```python
from build123d import *

# Parameters (mm, degrees)
SKIZZE1_W                                            = 33
SKIZZE1_H                                            = 20
SKIZZE1_W_2                                          = 13
SKIZZE1_H_2                                          = 13
AUFSATZ_LINEAR_AUSTRAGEN1_DEPTH                      = 10
STIRNSENKUNG_F_R_M4_ZYLINDERSCHRAUBE_MIT_D           = 4.5
STIRNSENKUNG_F_R_M4_ZYLINDERSCHRAUBE_MIT_CBORE_D     = 8
STIRNSENKUNG_F_R_M4_ZYLINDERSCHRAUBE_MIT_CBORE_DEPTH = 4.4
SKIZZE8_R                                            = 2.25
SCHNITT_LINEAR_AUSTRAGEN1_DEPTH                      = 11
M5_GEWINDEBOHRUNG1_D                                 = 4.2


with BuildPart() as part:
    # Skizze1 → Aufsatz-Linear austragen1 (new body)
    with BuildSketch(Plane.XY):
        Rectangle(SKIZZE1_W, SKIZZE1_H)
        Rectangle(SKIZZE1_W_2, SKIZZE1_H_2, mode=Mode.SUBTRACT)
    extrude(amount=AUFSATZ_LINEAR_AUSTRAGEN1_DEPTH)

    # Stirnsenkung für M4 Zylinderschraube mit Innensechskant1 (through all)
    with Locations(Plane.XY.offset(10)):
        with Locations((-11.5, 0)):
            CounterBoreHole(STIRNSENKUNG_F_R_M4_ZYLINDERSCHRAUBE_MIT_D / 2, STIRNSENKUNG_F_R_M4_ZYLINDERSCHRAUBE_MIT_CBORE_D / 2, STIRNSENKUNG_F_R_M4_ZYLINDERSCHRAUBE_MIT_CBORE_DEPTH)

    # Skizze8 → Schnitt-Linear austragen1 (cut, through all)
    with BuildSketch(Plane.XY.offset(10)):
        with Locations((-6.5, 6.5)):
            Circle(SKIZZE8_R)
        with Locations((-6.5, -6.5)):
            Circle(SKIZZE8_R)
        with Locations((6.5, -6.5)):
            Circle(SKIZZE8_R)
        with Locations((6.5, 6.5)):
            Circle(SKIZZE8_R)
    extrude(amount=-SCHNITT_LINEAR_AUSTRAGEN1_DEPTH, mode=Mode.SUBTRACT)

    # M5 Gewindebohrung1 (through all)
    with Locations(Plane.XY.offset(10)):
        with Locations((11.5, 0)):
            Hole(M5_GEWINDEBOHRUNG1_D / 2)


solid = part.part
```
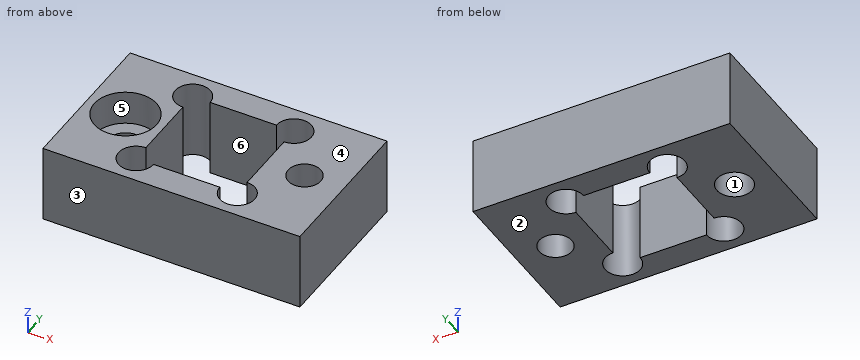
Model file for the job. Use its own axes, mm. Face numbers are marked on the shaded views. A direction names the side the tool comes from. Coordinates: 2 decimals unless noted, no trailing zeros. Order: outer loops, then holes, each group sorted by start corner. A loop starts at its lowest first (then second) coordinate and runs counter-clockwise, first axis right, second up. Notation, with made-up numbers: (22, -0.5) -> (48, -0.5) arc R8 cw to (48, 12.5) -> close; hole circle Ø10 at (-8, 31.5). An arc over 180 degrees is marked (long way). Answer as a JSON object with one key per item and string values. Group by question number.
1) Cut at A-A, the plane x = 11.5. Write the cut outline in (y, z).
2) Drill centre lines: L1, parallel to Y at x = 3.5, z = 0.5; L2, parallel to Y at x = 7.5, z = 5.5; L3, parallel to X at y = -7, z = 9.75. Where is each one in solid material? Low to high.
3) Cut at C-C, the plane y = 3.25. Write the cut outline in (x, z).
4) Flat gauge pins, fed straight in: pin 1 (2.5 mm diameter, centred on x = -12.5, y = -1.5, fed in from +Z); pin 2 (4 mm diameter, centred on x = 6.5, y = -6.5, fed in from -Z). Where does each tip first touch, or does it go through?
5) Which spindle directions (+Z, -Z, +X, -X, +Y, -Y) get a long thin tool onto all of the face, cutting with end or side? Do the marked faces 4, 5 and 6. Say none if no direction does.
6) Pull direction Y, two halves, no side cores. Call the marked faces 1, 2 and 3: +Y half, -Y half, draft (parallel to the pull), parting line (faces both ways), or undercut.
7) Cut at B-B, the plane z = 3.5. Write the cut outline in (x, y), then the cut area to 3 significant figures.
8) Cut at D-D, the plane x = -7. Write the cut outline in (y, z).
Check values:
{
 "1": {"outline": "(-10, 0) -> (-2.1, 0) -> (-2.1, 10) -> (-10, 10) -> close; (2.1, 0) -> (10, 0) -> (10, 10) -> (2.1, 10) -> close"},
 "2": {"L1": "y = -10 to -6.5, 6.5 to 10", "L2": "y = -10 to -8.52, -4.48 to 4.48, 8.52 to 10", "L3": "x = -16.5 to -8.69, -4.31 to 4.31, 8.69 to 16.5"},
 "3": {"outline": "(-16.5, 0) -> (-6.5, 0) -> (-6.5, 10) -> (-9.17, 10) -> (-9.17, 5.6) -> (-13.83, 5.6) -> (-13.83, 10) -> (-16.5, 10) -> close; (6.5, 0) -> (16.5, 0) -> (16.5, 10) -> (6.5, 10) -> close"},
 "4": {"pin 1": "stops at z = 5.6", "pin 2": "passes through"},
 "5": {"face 4": "+Z, +X, -X, +Y, -Y", "face 5": "+Z", "face 6": "+Z, -Z"},
 "6": {"face 1": "undercut", "face 2": "draft", "face 3": "-Y half"},
 "7": {"outline": "(-16.5, -10) -> (16.5, -10) -> (16.5, 10) -> (-16.5, 10) -> close; hole circle Ø4.5 at (-11.5, 0); hole (-6.5, -4.25) arc R2.25 ccw (long way) to (-4.25, -6.5) -> (4.25, -6.5) arc R2.25 ccw (long way) to (6.5, -4.25) -> (6.5, 4.25) arc R2.25 ccw (long way) to (4.25, 6.5) -> (-4.25, 6.5) arc R2.25 ccw (long way) to (-6.5, 4.25) -> close; hole circle Ø4.2 at (11.5, 0)", "area": "414 mm²"},
 "8": {"outline": "(-10, 0) -> (-8.69, 0) -> (-8.69, 10) -> (-10, 10) -> close; (-4.31, 0) -> (4.31, 0) -> (4.31, 10) -> (-4.31, 10) -> close; (8.69, 0) -> (10, 0) -> (10, 10) -> (8.69, 10) -> close"}
}
